```python
from build123d import *

# Parameters (mm, degrees)
SKETCH1_R           = 10
BOSS_EXTRUDE1_DEPTH = 493
SKETCH2_W           = 20
SKETCH2_H           = 20
SKETCH3_W           = 20
SKETCH3_H           = 20


with BuildPart() as part:
    # Sketch1 → Boss-Extrude1 (new body)
    with BuildSketch(Plane.XY):
        Circle(SKETCH1_R)
    extrude(amount=BOSS_EXTRUDE1_DEPTH)

    # Sketch2 → Revolve1 (revolve)
    with BuildSketch(Plane(origin=(0, 0, 0), x_dir=(0, 0, -1), z_dir=(1, 0, 0))):
        with Locations((-493, 0)):
            Rectangle(SKETCH2_W, SKETCH2_H)
    revolve(axis=Axis((0, 0, 528), (0, 1, 0)))

    # Sketch3 → Revolve2 (revolve)
    with BuildSketch(Plane(origin=(0, 0, 0), x_dir=(0, 0, -1), z_dir=(1, 0, 0))):
        Rectangle(SKETCH3_W, SKETCH3_H)
    revolve(axis=Axis((0, 0, -35), (0, 1, 0)))


solid = part.part
```
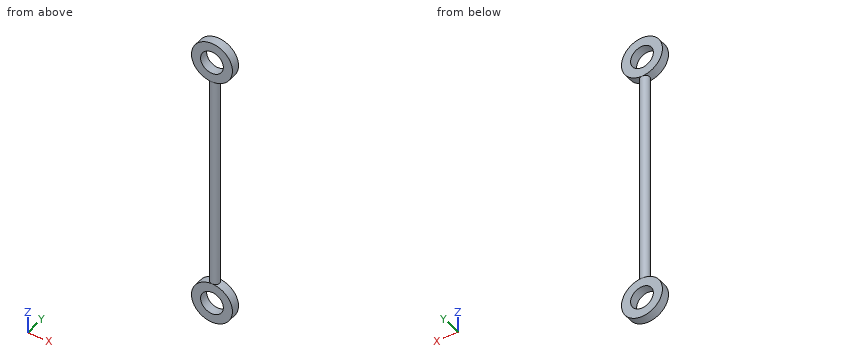
Verification items for the finished model (mm, model axes). Give positions to 0.01 mm unless a question says otherwise; leave off trailing zeros. Order: outer loops, then holes, each group sorted by start corner. A loop starts at its lowest first (then second) coordinate and runs counter-clockwise, first axis right, second up. Notation, with made-up numbers: (-8.75, 42) -> (44.25, 42) arc R11 cw to (44.25, 54) -> close; hole circle Ø7 at (49, 16). An arc over 180 degrees is marked (long way). One line per item, written item: value.
(1) Scan lines: line 1 along X through (y, z) = (-2.25, -35); line 2 along Z through (x, y) = (9.5, -2.5); line 3 along X through (y, z) = (-1.25, 266.5). Record each from-to range of solid material in increasing order. Write a range as [from, to].
Final values:
line 1: [-45, -25], [25, 45]
line 2: [-78.99, -58.12], [-11.88, 504.88], [551.12, 571.99]
line 3: [-9.92, 9.92]
(2) Sectioned sample at D-D on z = 72. Record the cut outline in (x, y), then the cut area to 3 significant figures.
Final values:
outline: circle Ø20 at (0, 0)
area: 314 mm^2
(3) Sectioned sample at A-A on z = 528. Record the cut outline in (x, y).
Final values:
outline: (-45, -10) -> (-25, -10) -> (-25, 10) -> (-45, 10) -> close; (25, -10) -> (45, -10) -> (45, 10) -> (25, 10) -> close
(4) Sectioned sample at B-B on y = 0. Record the cut outline in (x, z).
Final values:
outline: (-10, 8.87) arc R45 ccw (long way) to (10, 8.87) -> (10, 484.13) arc R45 ccw (long way) to (-10, 484.13) -> close; hole circle Ø50 at (0, -35); hole circle Ø50 at (0, 528)
(5) Sectioned sample at C-C on x = -35.5. Record the cut outline in (y, z), then the cut area to 3 significant figures.
Final values:
outline: (-10, -62.65) -> (10, -62.65) -> (10, -7.35) -> (-10, -7.35) -> close; (-10, 500.35) -> (10, 500.35) -> (10, 555.65) -> (-10, 555.65) -> close
area: 2,210 mm^2
(6) Gauge pin test, flat ends, axial feed: pin 1 (8 mm diameter, centred on y = 7.5, z = 79.5, fed in from +X); pin 2 (2 mm diameter, centred on x = 3.5, z = 217, fed in from -Y); pin 3 (1 mm diameter, centred on x = 14.5, y = -4.5, fed in from +Z). Record the tip position at first contact, or that the pin passes through.
Final values:
pin 1: x = 9.37
pin 2: y = -9.68
pin 3: z = 570.77
